Geometry check sheet. Reference: the model listing, model coordinates, mm. Face numbers are marked on the shaded views. A direction names the side the tool comes from. Give positions to 0.01 mm unless a question says otherwise; leave off trailing zeros. Write each loop counter-clockwise with the first axis right and the second up, starting at its lowest first coordinate (ties: lowest second). Pieces come first, ordered by that corner, then holes. Notation, with made-up numbers: M 51.25,80.5 L 103.25,80.5 A5 cw 103.25,85.5 Z; hole C -24.5,35.5 d9. An arc over 180 degrees is marked long. One line per item, written item: value. Start each with the question number.
1. Tool access check on the marked faces 1, 2 and 3. Record the directions out of +Z, -Z, +X, -X, +Y, -Y that give a thin tool (end or side, any length) a straight path to the whole face; none if there is none.
2. Release check for a two-part mould opening along X. For the marked faces 4, 5 and 6 record: pulls with the +X half, pulls with the -X half, needs draft (parallel to the pull), parting line crosses it, or undercut.
3. Gauge pin test, flat ends, axial feed: pin 1 (1 mm diameter, centred on y = -15.5, z = 28.5, fed in from -X); pin 2 (17.5 mm diameter, centred on x = 11.5, z = 24.5, fed in from -Y); pin 3 (1.5 mm diameter, centred on x = -19, z = 32.5, fed in from -Y); pin 4 (5 mm diameter, centred on x = -32, y = 3.5, fed in from -Z). Record the tip position at first contact, or that the pin passes through.
4. Scan lines: line 1 (Y direction, x = -41.5, z = 7); line 2 (X direction, y = -3.5, z = 11.5); line 3 (Z direction, x = 45.5, y = 18). Record each from-to range of solid material in increasing order.
5. Cross-section at D-D on z = 21. Record the cut outline in (x, y).
6. Cross-section at A-A on z = 10. Record the cut outline in (x, y), then the cut area to 3 significant figures.
7. Cross-section at C-C on x = -4. Record the cut outline in (y, z), then the cut area to 3 significant figures.
8. Cross-section at B-B on y = -6. Record the cut outline in (x, z).
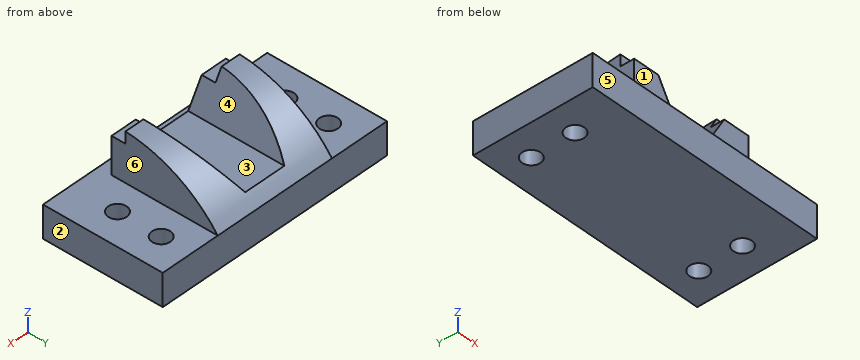
from build123d import *

# Parameters (mm, degrees)
SKETCH1_W           = 106
SKETCH1_H           = 52
BOSS_EXTRUDE1_DEPTH = 14
SKETCH2_R           = 4
CUT_EXTRUDE1_DEPTH  = 14
BOSS_EXTRUDE2_DEPTH = 27
CUT_EXTRUDE2_DEPTH  = 79.485834959


with BuildPart() as part:
    # Sketch1 → Boss-Extrude1 (new body)
    with BuildSketch(Plane.XY):
        Rectangle(SKETCH1_W, SKETCH1_H)
    extrude(amount=BOSS_EXTRUDE1_DEPTH)

    # Sketch2 → Cut-Extrude1 (cut)
    with BuildSketch(Plane.XY.offset(14)):
        with Locations((39.576420428, 13)):
            Circle(SKETCH2_R)
        with Locations((39.576420428, -6)):
            Circle(SKETCH2_R)
    cut_extrude1 = extrude(amount=-CUT_EXTRUDE1_DEPTH, mode=Mode.SUBTRACT)

    # Mirror1: Cut-Extrude1 across plane
    add(cut_extrude1.mirror(Plane.ZY), mode=Mode.SUBTRACT)

    # Sketch4 → Boss-Extrude2 (add, symmetric)
    with BuildSketch(Plane.ZY):
        with BuildLine():
            Line((14, 26), (14, -20.108852612))
            Line((14, -20.108852612), (30, -20.108852612))
            Line((30, -20.108852612), (30, -14.108852612))
            Line((30, -14.108852612), (35, -14.108852612))
            ThreePointArc((35, -14.108852612), (28.906357886, 8.252633347), (14, 26))
        make_face()
    extrude(amount=BOSS_EXTRUDE2_DEPTH, both=True)

    # Sketch6 → Cut-Extrude2 (cut, through all)
    with BuildSketch(Plane.XZ.offset(20.108852612)):
        Polygon((-9.237604307, 19), (-18.475208614, 35), (18.475208614, 35), (9.237604307, 19), align=None)
    extrude(amount=-CUT_EXTRUDE2_DEPTH, mode=Mode.SUBTRACT)


solid = part.part
Report:
1. face 1: +Z, +X, -X, -Y
1. face 2: +Z, -Z, +X, +Y, -Y
1. face 3: +Z, +Y, -Y
2. face 4: undercut
2. face 5: needs draft
2. face 6: pulls with the +X half
3. pin 1: stops at x = -27
3. pin 2: stops at y = -20.11
3. pin 3: stops at y = -14.11
3. pin 4: stops at z = 0
4. line 1: y = -26 to -9.51, -2.49 to 9.49, 16.51 to 26
4. line 2: x = -53 to -42.7, -36.45 to 36.45, 42.7 to 53
4. line 3: z = 0 to 14
5. outline: M -27,-20.11 L -10.39,-20.11 L -10.39,19.56 L -27,19.56 Z; M 10.39,-20.11 L 27,-20.11 L 27,19.56 L 10.39,19.56 Z
6. outline: M -53,-26 L 53,-26 L 53,26 L -53,26 Z; hole C -39.58,-6 d8; hole C -39.58,13 d8; hole C 39.58,-6 d8; hole C 39.58,13 d8
6. area: 5,310 mm^2
7. outline: M -26,0 L 26,0 L 26,14 A54 ccw 21.64,19 L -20.11,19 L -20.11,14 L -26,14 Z
7. area: 948 mm^2
8. outline: M -53,0 L -43.58,0 L -43.58,14 L -53,14 Z; M -35.58,0 L 35.58,0 L 35.58,14 L 27,14 L 27,33.98 L 17.88,33.98 L 9.24,19 L -9.24,19 L -17.88,33.98 L -27,33.98 L -27,14 L -35.58,14 Z; M 43.58,0 L 53,0 L 53,14 L 43.58,14 Z
